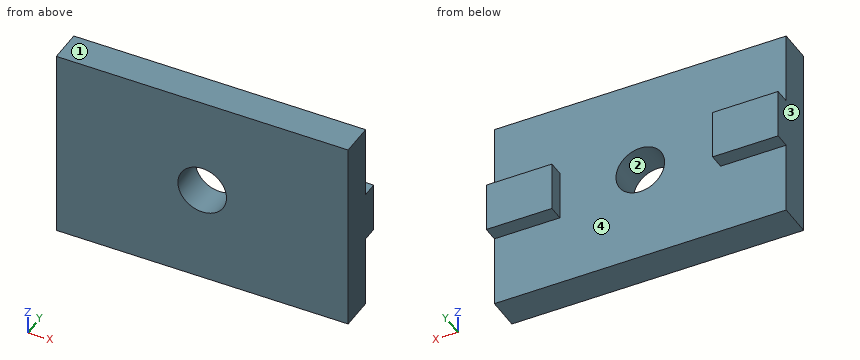
from build123d import *

# Parameters (mm, degrees)
SKETCH1_W           = 38.1
SKETCH1_H           = 25.4
SKETCH1_R           = 3.175
BOSS_EXTRUDE1_DEPTH = 4.35
SKETCH2_W           = 8.5598
SKETCH2_H           = 6.476913764
BOSS_EXTRUDE2_DEPTH = 2


with BuildPart() as part:
    # Sketch1 → Boss-Extrude1 (new body)
    with BuildSketch(Plane(origin=(0, 0, 0), x_dir=(1, 0, 0), z_dir=(0, 1, 0))):
        with Locations((16.172116278, 18.931628639)):
            Rectangle(SKETCH1_W, SKETCH1_H)
        with Locations(Location((16.172116278, 18.931628639, 0), (0, 0, 270))):
            Circle(SKETCH1_R, mode=Mode.SUBTRACT)
    extrude(amount=BOSS_EXTRUDE1_DEPTH)

    # Sketch2 → Boss-Extrude2 (add)
    with BuildSketch(Plane(origin=(0, 4.35, 0), x_dir=(1, 0, 0), z_dir=(0, 1, 0))):
        with Locations((1.402016278, 18.931628639)):
            Rectangle(SKETCH2_W, SKETCH2_H)
        with Locations((30.942216278, 18.931628639)):
            Rectangle(SKETCH2_W, SKETCH2_H)
    extrude(amount=BOSS_EXTRUDE2_DEPTH)


solid = part.part
Work out the finished part from the listing and answer in its coordinate system (mm). Face numbers are marked on the shaded views. Coordinates: 2 decimals unless noted, no trailing zeros. Loops run counter-clockwise (first coordinate to the right, second up) from the corner with the lowest first, then second, coordinate; pieces in that order, holes last. Notation, with made-up numbers: (25, -15) -> (34, -15) arc R11 ccw to (34, -11) -> close; hole circle Ø7 at (0.5, 64). An arc over 180 degrees is marked (long way). Write each question's results on one line, items separated by ' | '. Start each with the question number.
1) Consider line 1 along Y through (x, z) = (1, -22.75); line 2 along Z through (x, y) = (27, 5); line 3 along Z through (x, y) = (14, 2.5). Determine where each line is inside the solid, lowest interval first.
2) Flat-ended cylindrical pins translate along their axes: P1, Ø1.6, axis at x = 33, y = 5.5, coming from the +Z side; P2, Ø0.6, axis at x = 29, y = 5.5, coming from the -Z side. Find the tip coordinate at first contact, or state that the pin passes through.
3) Find section A-A on y = 4.75. Determine the outline of the cut face in (x, z).
4) The mould has two halves that part along X. Classify the marked faces 1, 2, 3 and 4: pulls with the +X half, pulls with the -X half, needs draft (parallel to the pull), parting line crosses it, or undercut.
5) Find section D-D on z = -29.25. Determine the outline of the cut face in (x, y), then the cut area to 3 significant figures.
6) Find section C-C on z = -19. Determine the outline of the cut face in (x, y).
7) Find section B-B on x = 4.5. Determine the outline of the cut face in (y, z), then the cut area to 3 significant figures.
Response values:
1) line 1: y = 0 to 4.35 | line 2: z = -22.17 to -15.69 | line 3: z = -31.63 to -21.25, -16.62 to -6.23
2) P1: stops at z = -15.69 | P2: stops at z = -22.17
3) outline: (-2.88, -22.17) -> (5.68, -22.17) -> (5.68, -15.69) -> (-2.88, -15.69) -> close; (26.66, -22.17) -> (35.22, -22.17) -> (35.22, -15.69) -> (26.66, -15.69) -> close
4) face 1: needs draft | face 2: undercut | face 3: pulls with the -X half | face 4: undercut
5) outline: (-2.88, 0) -> (35.22, 0) -> (35.22, 4.35) -> (-2.88, 4.35) -> close | area: 166 mm^2
6) outline: (-2.88, 0) -> (13, 0) -> (13, 4.35) -> (5.68, 4.35) -> (5.68, 6.35) -> (-2.88, 6.35) -> close; (19.35, 0) -> (35.22, 0) -> (35.22, 6.35) -> (26.66, 6.35) -> (26.66, 4.35) -> (19.35, 4.35) -> close
7) outline: (0, -31.63) -> (4.35, -31.63) -> (4.35, -22.17) -> (6.35, -22.17) -> (6.35, -15.69) -> (4.35, -15.69) -> (4.35, -6.23) -> (0, -6.23) -> close | area: 123 mm^2
